Check sheet for the modelled part. Datum: model origin and axes. Units: mm. A direction names the side the tool comes from. Round coordinates to 2 decimals unless told otherwise and drop trailing zeros. Write each loop counter-clockwise with the first axis right and the second up, starting at its lowest first coordinate (ties: lowest second). Pieces come first, ordered by that corner, then holes. Notation, with made-up numbers: (34.5, -13.5) - (87.5, -13.5) arc R9 ccw to (87.5, -5.5) - close; hole circle Ø11 at (30.5, 87). An arc over 180 degrees is marked (long way). Use one line per item in the form item = value. Start each with the question number.
1) Set-up check for faces 4 (the face through (30, -15, 15)), 5 (the face through (15.161, -27.199, 2.785)): record each of +Z, -Z, +X, -X, +Y, -Y from which the full face is reachable in a straight line by a thin tool's end or side.
2) Scan lines: probe 1 along X at (y, z) = (-25.5, 11.25); probe 2 along Y at (x, z) = (10.5, 24.5). Record each from-to range of solid material in increasing order.
3) Section check C-C (x = 24.25). Record the boundary of the cut face in (y, z), then the cut area to 3 significant figures.
4) Draft check along X on faces 1 (the face through (2.785, -27.199, 15.161)), 2 (the face through (29.715, -29.699, 15.196)), 3 (the face through (15.196, -0.301, 0.285)). Enter one of: +X half, -X half, draft (parallel to the pull), parting line (faces both ways), or undercut.
5) Section check A-A (y = -15). Record the boundary of the cut face in (x, z), then the cut area to 3 significant figures.
6) Section check B-B (z = 14). Record the boundary of the cut face in (x, y), then the cut area to 3 significant figures.
from build123d import *

# Parameters (mm, degrees)
F0_W     = 30
F0_H     = 30
F1_DEPTH = 30
F2_T     = -2.5
F3_R     = 1


with BuildPart() as f1:
    # F0 (on Front) → F1 (new body)
    with BuildSketch(Plane.XZ):
        with Locations((15, 15)):
            Rectangle(F0_W, F0_H)
    extrude(amount=F1_DEPTH)

    # F2
    f2_openings = [f1.faces().sort_by_distance(p)[0] for p in [
        (15, 0, 15),
    ]]
    offset(amount=F2_T, openings=f2_openings)

    # F3
    f3_edges = [f1.edges().sort_by_distance(p)[0] for p in [
        (30, -15, 30),
        (0, -15, 30),
        (30, -15, 0),
        (2.5, -13.75, 2.5),
        (0, 0, 15),
        (15, 0, 0),
        (15, -30, 0),
        (15, 0, 30),
        (15, -30, 30),
        (0, -30, 15),
        (30, 0, 15),
        (30, -30, 15),
        (27.5, -13.75, 2.5),
        (2.5, -13.75, 27.5),
        (27.5, -13.75, 27.5),
        (15, 0, 2.5),
        (15, -27.5, 2.5),
        (15, 0, 27.5),
        (15, -27.5, 27.5),
        (2.5, 0, 15),
        (2.5, -27.5, 15),
        (27.5, 0, 15),
        (27.5, -27.5, 15),
        (0, -15, 0),
    ]]
    fillet(f3_edges, radius=F3_R)


solid = f1.part
Results are:
q1.face_4 = +Z, -Z, +X, +Y, -Y
q1.face_5 = +Y
q2.probe_1 = 0 to 2.5, 27.5 to 30
q2.probe_2 = -30 to -27.5
q3.outline = (-30, 1) arc R1 ccw to (-29, 0) - (-1, 0) arc R1 ccw to (0, 1) - (0, 1.5) arc R1 ccw to (-1, 2.5) - (-26.5, 2.5) arc R1 cw to (-27.5, 3.5) - (-27.5, 26.5) arc R1 cw to (-26.5, 27.5) - (-1, 27.5) arc R1 ccw to (0, 28.5) - (0, 29) arc R1 ccw to (-1, 30) - (-29, 30) arc R1 ccw to (-30, 29) - close
q3.area = 212 mm²
q4.face_1 = undercut
q4.face_2 = +X half
q4.face_3 = draft
q5.outline = (0, 1) arc R1 ccw to (1, 0) - (29, 0) arc R1 ccw to (30, 1) - (30, 29) arc R1 ccw to (29, 30) - (1, 30) arc R1 ccw to (0, 29) - close; hole (2.5, 3.5) arc R1 ccw to (3.5, 2.5) - (26.5, 2.5) arc R1 ccw to (27.5, 3.5) - (27.5, 26.5) arc R1 ccw to (26.5, 27.5) - (3.5, 27.5) arc R1 ccw to (2.5, 26.5) - close
q5.area = 275 mm²
q6.outline = (0, -29) arc R1 ccw to (1, -30) - (29, -30) arc R1 ccw to (30, -29) - (30, -1) arc R1 ccw to (29, 0) - (28.5, 0) arc R1 ccw to (27.5, -1) - (27.5, -26.5) arc R1 cw to (26.5, -27.5) - (3.5, -27.5) arc R1 cw to (2.5, -26.5) - (2.5, -1) arc R1 ccw to (1.5, 0) - (1, 0) arc R1 ccw to (0, -1) - close
q6.area = 212 mm²
